```python
from build123d import *

# Parameters (mm, degrees)
F1_DEPTH = 25


with BuildPart() as f1:
    # F0 (on Top) → F1 (new body)
    with BuildSketch(Plane.XY):
        Polygon((21.36452, 29.405739), (-21.36452, 29.405739), (-34.56852, -11.231993), (0, -36.347493), (34.56852, -11.231993), align=None)
    extrude(amount=F1_DEPTH)

    # F1_face (on face) → F4 section 0
    with BuildSketch(Plane.XY.offset(25), mode=Mode.PRIVATE) as f4_s0:
        Polygon((34.56852, -11.231993), (21.36452, 29.405739), (-21.36452, 29.405739), (-34.56852, -11.231993), (0, -36.347493), align=None)
    loft([f4_s0.sketch, Vertex(0, 0, 150)])


solid = f1.part
```
Geometry check sheet. Reference: the model listing, model coordinates, mm. Coordinates: 2 decimals unless noted, no trailing zeros. Order: outer loops, then holes, each group sorted by start corner. A loop starts at its lowest first (then second) coordinate and runs counter-clockwise, first axis right, second up. Notation, with made-up numbers: (73.25, 23.25) - (114.25, 23.25) arc R23 ccw to (114.25, 33.25) - close; hole circle Ø7 at (-7.5, -5). An arc over 180 degrees is marked (long way). Use one line per item in the form item = value.
1. Scan lines: line 1 (Y direction, x = 14.5, z = 60); line 2 (Y direction, x = 14.5, z = 42); line 3 (X direction, y = -9, z = 73). Record each from-to range of solid material in increasing order.
Here are the results:
line_1 = -15.64 to 21.17
line_2 = -20.87 to 25.41
line_3 = -18.43 to 18.43
2. Section check D-D (z = 117). Record the boundary of the cut face in (x, y), then the cut area to 3 significant figures.
Here are the results:
outline = (-9.13, -2.97) - (0, -9.6) - (9.13, -2.97) - (5.64, 7.76) - (-5.64, 7.76) - close
area = 219 mm²
3. Section check C-C (x = -6). Record the boundary of the cut face in (y, z), then the cut area to 3 significant figures.
Here are the results:
outline = (-31.99, 0) - (29.41, 0) - (29.41, 25) - (8.26, 114.9) - (-1.95, 128.3) - (-31.99, 25) - close
area = 5,020 mm²
4. Section check B-B (z = 12.5). Record the boundary of the cut face in (x, y), then the cut area to 3 significant figures.
Here are the results:
outline = (-34.57, -11.23) - (0, -36.35) - (34.57, -11.23) - (21.36, 29.41) - (-21.36, 29.41) - close
area = 3,140 mm²
5. Section check A-A (y = -7.5). Record the boundary of the cut face in (x, z), then the cut area to 3 significant figures.
Here are the results:
outline = (-33.36, 0) - (33.36, 0) - (33.36, 25) - (23.08, 66.53) - (0, 124.21) - (-23.08, 66.53) - (-33.36, 25) - close
area = 5,340 mm²
6. Gauge pin test, flat ends, axial feed: pin 1 (5 mm diameter, centred on x = 10, z = 82.5, fed in from +Y); pin 2 (1.5 mm diameter, centred on y = 17.5, z = 40, fed in from +X); pin 3 (5 mm diameter, centred on y = -5, z = 104.5, fed in from +X). Record the tip position at first contact, or that the pin passes through.
Here are the results:
pin_1 = 16.47
pin_2 = 21.83
pin_3 = 13.25
